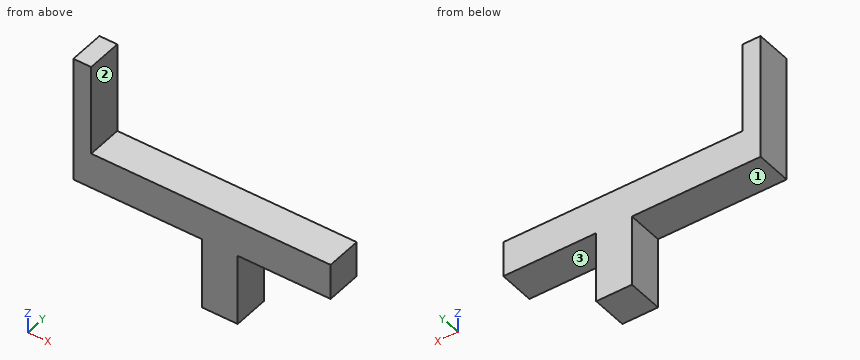
```python
from build123d import *

# Parameters (mm, degrees)
SKETCH_W     = 10
SKETCH_H     = 10
PAD_DEPTH    = 30
SKETCH001_W  = 10
SKETCH001_H  = 10
PAD001_DEPTH = 26
SKETCH002_W  = 10
SKETCH002_H  = 10
PAD002_DEPTH = 36
SKETCH003_W  = 5
SKETCH003_H  = 10
PAD003_DEPTH = 25.4


with BuildPart() as part:
    # Sketch → Pad (new body)
    with BuildSketch(Plane.XY):
        with Locations((5, 5)):
            Rectangle(SKETCH_W, SKETCH_H)
    extrude(amount=PAD_DEPTH)

    # Sketch001 (on Face2 of Pad) → Pad001 (join)
    with BuildSketch(Plane.YZ.offset(10)):
        with Locations((5, 25)):
            Rectangle(SKETCH001_W, SKETCH001_H)
    extrude(amount=PAD001_DEPTH)

    # Sketch002 (on Face3 of Pad001) → Pad002 (join)
    with BuildSketch(Plane(origin=(0, 0, 0), x_dir=(0, -1, 0), z_dir=(-1, 0, 0))):
        with Locations((-5, 25)):
            Rectangle(SKETCH002_W, SKETCH002_H)
    extrude(amount=PAD002_DEPTH)

    # Sketch003 (on Face10 of Pad002) → Pad003 (join)
    with BuildSketch(Plane.XY.offset(30)):
        with Locations((-33.5, 5)):
            Rectangle(SKETCH003_W, SKETCH003_H)
    extrude(amount=PAD003_DEPTH)


solid = part.part
```
Can you work these out from the model? Positions are in its coordinate system, mm. Face numbers are marked on the shaded views. A direction names the side the tool comes from. Coordinates: 2 decimals unless noted, no trailing zeros. Loops run counter-clockwise (first coordinate to the right, second up) from the corner with the lowest first, then second, coordinate; pieces in that order, holes last.
1) Imagine slicing it at C-C on z = 3.5. List the corners of the cut face in (x, y) for me, plus the area to 3 significant figures.
2) For pin 1 (3 mm diameter, centred on x = 15, y = 8, fed in from -Z); pin 2 (5 mm diameter, centred on y = 7, z = 8, fed in from -X), each with a flat end and sliding along its axis, tell me the tip position at first contact or that it passes through.
3) Imagine slicing it at A-A on y = 6. List the corners of the cut face in (x, z) for me, plus the area to 3 significant figures.
4) I need wall thicknesses on probe 1 along Z at (x, y) = (-22, 0.75); probe 2 along X at (y, z) = (4.25, 18); probe 3 along X at (y, z) = (1.5, 40). Which ranges of each line are inside material? Lowest first, please.
5) Which directions (+Z, -Z, +X, -X, +Y, -Y) give clear straight access to the entire face, cutting with the end or side of a thin tool? Please do the marked faces 1, 2 and 3.
6) Imagine slicing it at B-B on x = 4. List the corners of the cut face in (y, z) for me, plus the area to 3 significant figures.
Completed:
1. outline: (0, 0) - (10, 0) - (10, 10) - (0, 10) - close
1. area: 100 mm2
2. pin 1: stops at z = 20
2. pin 2: stops at x = 0
3. outline: (-36, 20) - (0, 20) - (0, 0) - (10, 0) - (10, 20) - (36, 20) - (36, 30) - (-31, 30) - (-31, 55.4) - (-36, 55.4) - close
3. area: 1,050 mm2
4. probe 1: z = 20 to 30
4. probe 2: x = 0 to 10
4. probe 3: x = -36 to -31
5. face 1: -Z, -X, +Y, -Y
5. face 2: +Z, +X, +Y, -Y
5. face 3: -Z, +X, +Y, -Y
6. outline: (0, 0) - (10, 0) - (10, 30) - (0, 30) - close
6. area: 300 mm2
